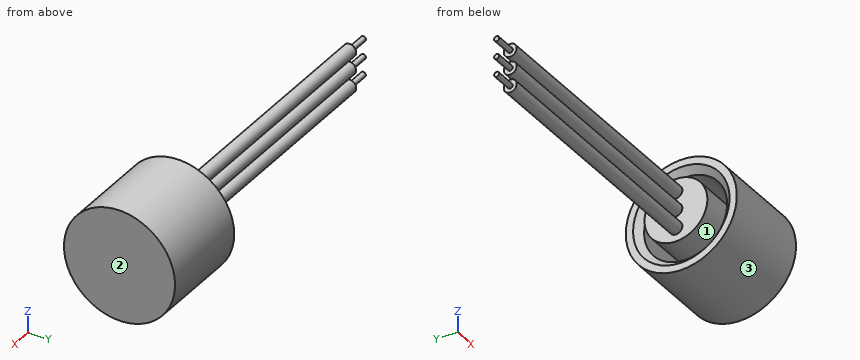
```python
from build123d import *


with BuildPart() as part:
    # Sketch1 → Revolve1 (revolve)
    with BuildSketch(Plane.XY.offset(-0.0942096)):
        Polygon((35.6108, -12.191773113), (35.6108, -5.080397281), (54.6608, -5.080396955), (54.6608, -2.794255147), (39.0398, -2.794245161), (37.5158, -1.270188911), (37.5158, 0.380874088), (58.4708, 0.380865578), (58.4708, -12.191773113), align=None)
    revolve(axis=Axis((58.4708, -12.191773113, -0.0942096), (-1, 0, 0)))

    # Sketch2 → Revolve2 (revolve)
    with BuildSketch(Plane(origin=(0, -12.191772951, 0), x_dir=(1, 0, 0), z_dir=(0, 1, 0))):
        Polygon((-27.8892, -3.9697904), (-27.8892, -3.3982904), (-23.0632, -3.3982904), (-23.0632, -2.509290489), (35.6108, -2.509290489), (35.6108, -3.9697904), align=None)
    revolve(axis=Axis((35.6108, -12.191772951, 3.9697904), (-1, 0, 0)))

    # Sketch3 → Revolve3 (revolve)
    with BuildSketch(Plane(origin=(0, -12.191772951, 0), x_dir=(1, 0, 0), z_dir=(0, 1, 0))):
        Polygon((-27.8892, 4.1582096), (-27.8892, 4.7297096), (-23.0632, 4.7297096), (-23.0632, 5.618709512), (35.6108, 5.618709512), (35.6108, 4.1582096), align=None)
    revolve(axis=Axis((35.6108, -12.191772951, -4.1582096), (-1, 0, 0)))

    # Sketch4 → Revolve4 (revolve)
    with BuildSketch(Plane(origin=(0, -12.191772951, 0), x_dir=(1, 0, 0), z_dir=(0, 1, 0))):
        Polygon((-27.8892, 0.0942096), (-27.8892, 0.6657096), (-23.0632, 0.6657096), (-23.0632, 1.554709511), (35.6108, 1.554709511), (35.6108, 0.0942096), align=None)
    revolve(axis=Axis((35.6108, -12.191772951, -0.0942096), (-1, 0, 0)))


solid = part.part
```
Source: CAD feature listing. Evaluate the final solid. Frame: model axes, mm. Face numbers are marked on the shaded views. Round coordinates to 2 decimals unless told otherwise and drop trailing zeros. Loops run counter-clockwise (first coordinate to the right, second up) from the corner with the lowest first, then second, coordinate; pieces in that order, holes last. Notation, with made-up numbers: M -1,-38.75 L 25,-38.75 A23 cw 25,-20.75 Z; hole C 82,27 d1. An arc over 180 degrees is marked long. Use a Markdown table: item, result. Add a question column.
1. Section query B-B on x = 10. Return the cut outline in (y, z).
2. Line query: line 1 (Z direction, x = 41.5, y = -12); line 2 (Z direction, x = 42, y = -17); line 3 (Y direction, x = 39.5, z = 0.25). Output: solid intervals per line, ascending.
3. Mould query, pull axis Z, two halves, no side actions, for the marked faces 1, 2 and 3. Classes: pulls with the +Z half, pulls with the -Z half, needs draft (parallel to the pull), parting line crosses it, or undercut.
4. Section query A-A on x = 52.5. Return the cut outline in (y, z), then the cut area to 3 significant figures.
5. Contact query for flat-ended pins moving along their axis: P1, Ø0.9, axis at y = -12, z = -1, coming from the -X side; P2, Ø2, axis at x = 39, z = 4, coming from the -Y side; P3, Ø1.5, axis at x = -11.5, z = 4.5, coming from the -Y side; P4, Ø3, axis at x = 49.5, y = -8.5, coming from the -Z side. Output: stop coordinate, or through.
Reported:
| question | item | result |
|---|---|---|
| 1 | outline | C -12.19,-4.16 d2.92; C -12.19,-0.09 d2.92; C -12.19,3.97 d2.92 |
| 2 | line 1 | z = -12.67 to -9.49, -7.2 to 7.01, 9.3 to 12.48 |
| 2 | line 2 | z = -11.71 to -8.17, -5.33 to 5.15, 7.98 to 11.52 |
| 2 | line 3 | y = -24.76 to -21.58, -19.29 to -5.09, -2.8 to 0.38 |
| 3 | face 1 | undercut |
| 3 | face 2 | needs draft |
| 3 | face 3 | parting line crosses it |
| 4 | outline | C -12.19,-0.09 d25.15; C -12.19,-0.09 d14.22; hole C -12.19,-0.09 d18.8 |
| 4 | area | 378 mm² |
| 5 | P1 | stops at x = -27.89 |
| 5 | P2 | stops at y = -24.38 |
| 5 | P3 | stops at y = -13.65 |
| 5 | P4 | stops at z = -12.47 |
